Can you work these out from the model? Positions are in its coordinate system, mm. Face numbers are marked on the shaded views. A direction names the side the tool comes from. Give positions to 0.01 mm unless a question says otherwise; leave off trailing zeros. Order: outer loops, then holes, each group sorted by start corner. A loop starts at its lowest first (then second) coordinate and runs counter-clockwise, first axis right, second up. Notation, with made-up numbers: (8.25, 14) -> (49.25, 14) arc R27 ccw to (49.25, 47) -> close; hole circle Ø11 at (-19.5, -32.75). An arc over 180 degrees is marked (long way). Answer as a JSON object with one key per item and string values.
```python
from build123d import *

# Parameters (mm, degrees)
F0_W     = 5.4636245876
F0_H     = 33.2398892505
F1_DEPTH = 2.54
F2_DEPTH = 25.4
F4_DEPTH = 125.8997323481
F5_DEPTH = 125.8997323481
F6_W     = 22.352
F6_H     = 49.1605467501
F7_DEPTH = 125.8997323481


with BuildPart() as f1:
    # F0 (on Front) → F1 (new body)
    with BuildSketch(Plane.XZ):
        with BuildLine():
            ThreePointArc((-58.7834570181, -20.4847763815), (-61.356974344, -57.1489152116), (-24.6143243603, -58.0761367374))
            Line((-24.6143243603, -58.0761367374), (21.8259629316, -20.4486662023))
            Line((21.8259629316, -20.4486662023), (19.6400941384, -18.2968238675))
            Line((19.6400941384, -18.2968238675), (-26.6574493018, -55.8086385705))
            ThreePointArc((-26.6574493018, -55.8086385705), (-59.1008466393, -55.0994768945), (-56.7221636318, -22.7356265638))
            Line((-56.7221636318, -22.7356265638), (-16.9208807766, 17.6950224269))
            Line((-16.9208807766, 17.6950224269), (-19.0929825471, 19.8333120442))
            Line((-19.0929825471, 19.8333120442), (-58.7834570181, -20.4847763815))
        make_face()
        with BuildLine():
            Line((-26.6574493018, -55.8086385705), (19.6400941384, -18.2968238675))
            Line((19.6400941384, -18.2968238675), (-16.9208807766, 17.6950224269))
            Line((-16.9208807766, 17.6950224269), (-56.7221636318, -22.7356265638))
            ThreePointArc((-56.7221636318, -22.7356265638), (-59.1008466393, -55.0994768945), (-26.6574493018, -55.8086385705))
        make_face()
        with Locations((-45.2741895661, -38.6369622716)):
            Rectangle(F0_W, F0_H, mode=Mode.SUBTRACT)
    extrude(amount=F1_DEPTH)

    # F0 (on Front) → F2 (join)
    with BuildSketch(Plane.XZ):
        with BuildLine():
            Line((19.6400941384, -18.2968238675), (21.8259629316, -20.4486662023))
            Line((21.8259629316, -20.4486662023), (63.3089077462, 13.162200025))
            ThreePointArc((63.3089077462, 13.162200025), (65.3407579963, 57.9152109511), (20.5974919239, 60.1514004699))
            Line((20.5974919239, 60.1514004699), (-19.0929825471, 19.8333120442))
            Line((-19.0929825471, 19.8333120442), (-16.9208807766, 17.6950224269))
            Line((-16.9208807766, 17.6950224269), (22.703735232, 57.9462109895))
            ThreePointArc((22.703735232, 57.9462109895), (63.0846270143, 55.8657762462), (61.315579372, 15.4700450325))
            Line((61.315579372, 15.4700450325), (19.6400941384, -18.2968238675))
        make_face()
        with BuildLine():
            Line((-16.9208807766, 17.6950224269), (19.6400941384, -18.2968238675))
            Line((19.6400941384, -18.2968238675), (61.315579372, 15.4700450325))
            ThreePointArc((61.315579372, 15.4700450325), (63.0846270143, 55.8657762462), (22.703735232, 57.9462109895))
            Line((22.703735232, 57.9462109895), (-16.9208807766, 17.6950224269))
        make_face()
    extrude(amount=F2_DEPTH)

    # F3 (on face) → F4 (cut, through all)
    with BuildSketch(Plane(origin=(-19.611689488, 0, 19.306402941), x_dir=(0, -1, 0), z_dir=(-0.7126316385, 0, 0.7015384151))):
        Polygon((25.4, 57.3157229122), (2.54, 0.7393849428), (25.4, 0.7393849428), align=None)
    extrude(amount=-F4_DEPTH, mode=Mode.SUBTRACT)

    # F3 (on face) → F5 (cut, through all)
    with BuildSketch(Plane(origin=(-19.611689488, 0, 19.306402941), x_dir=(0, -1, 0), z_dir=(-0.7126316385, 0, 0.7015384151))):
        Polygon((0, 1.9966368976), (22.352, 57.3157229122), (0, 57.3157229122), align=None)
    extrude(amount=-F5_DEPTH, mode=Mode.SUBTRACT)

    # F6 (on face) → F7 (cut, through all)
    with BuildSketch(Plane(origin=(-19.611689488, 0, 19.306402941), x_dir=(0, -1, 0), z_dir=(-0.7126316385, 0, 0.7015384151))):
        with Locations((11.176, 81.8959962873)):
            Rectangle(F6_W, F6_H)
    extrude(amount=-F7_DEPTH, mode=Mode.SUBTRACT)


solid = f1.part
```
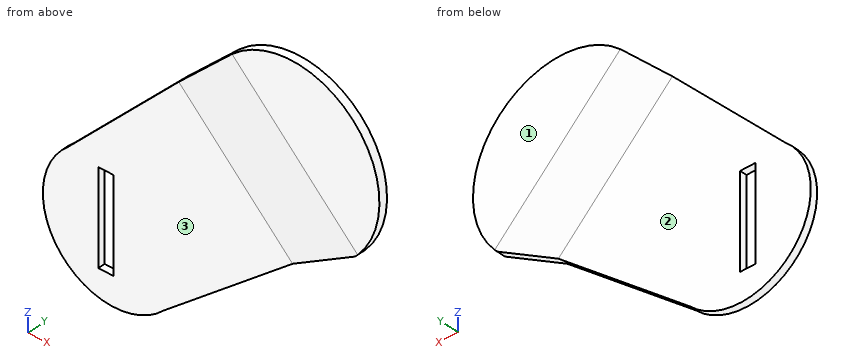
1. If we section it at B-B on x = -5: Please give me the cut outline in (y, z), then the cut area to 3 significant figures.
Worked answers:
{"outline": "(-10.66, 34.15) -> (-2.54, 5.96) -> (-2.54, -42.18) -> (0, -42.18) -> (0, 7.72) -> (-7.61, 34.15) -> close", "area": "208 mm²"}
2. If we section it at A-A on z = -30: Please give me the cut outline in (x, y), then the cut area to 3 significant figures.
Worked answers:
{"outline": "(-65.9, -2.54) -> (-48.01, -2.54) -> (-48.01, 0) -> (-65.9, 0) -> close; (-42.54, -2.54) -> (10.04, -2.54) -> (10.04, 0) -> (-42.54, 0) -> close", "area": "179 mm²"}
3. Please list where these lines run through material, in increasing order: L1, parallel to Y at x = -28, z = -31.5; L2, parallel to X at y = -2.5, z = -59; L3, parallel to Y at x = 45.5, z = 1.
Worked answers:
{"L1": "-2.54 to 0", "L2": "-59.49 to -25.59", "L3": "-15.43 to -12.38"}
4. Will these pins go through, and if not, where does the flat tip stop? pin 1 Ø1.3 at (x, y) = (-46, -1.5) entering from -Z; pin 2 Ø2 at (x, z) = (40.5, 4.5) entering from +Y; pin 3 Ø5 at (x, z) = (51.5, 4.5) entering from +Y.
Worked answers:
{"pin 1": "z = -65.32", "pin 2": "y = -11.57", "pin 3": "y = -14.08"}
5. If we section it at C-C on z = 57.5: Please give me the cut outline in (x, y), then the cut area to 3 significant figures.
Worked answers:
{"outline": "(17.99, -23.9) -> (23.29, -25.4) -> (65.71, -25.4) -> (65.71, -22.35) -> (23.29, -22.35) -> (17.99, -20.85) -> close", "area": "145 mm²"}
6. If we section it at D-D on y = -16: Please give me the cut outline in (x, z), then the cut area to 3 significant figures.
Worked answers:
{"outline": "(4.28, 43.57) -> (47.87, 0.66) -> (53.77, 5.43) -> (9.57, 48.95) -> close", "area": "465 mm²"}
7. For the marked faces 1, 2 and 3, which set-ups out of +Z, -Z, +X, -X, +Y, -Y let a thin tool reach every point of the face, with its end or its side?
Worked answers:
{"face 1": "+Z, +X, +Y", "face 2": "+Z, -Z, +X, -X, +Y", "face 3": "-Z, -X, -Y"}
